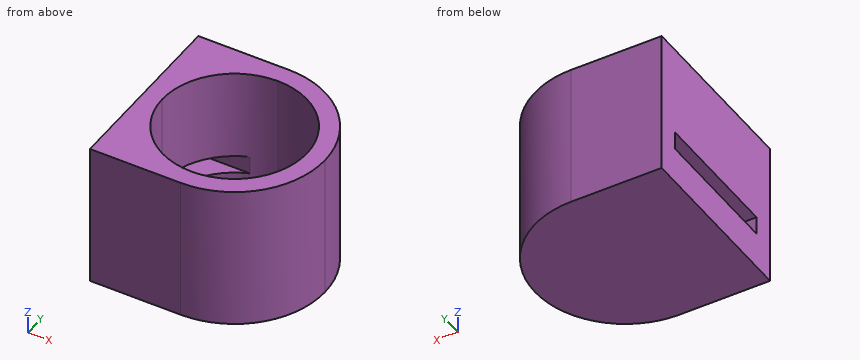
from build123d import *

# Parameters (mm, degrees)
F1_DEPTH = 25.4
F2_R     = 12.7
F3_DEPTH = 3.175
F5_DEPTH = 12.7


with BuildPart() as f1:
    # F0 (on Top) → F1 (new body)
    with BuildSketch(Plane.XY):
        with BuildLine():
            ThreePointArc((-15.875, 0), (-11.2253201513, 11.2253201513), (0, 15.875))
            Line((0, 15.875), (-15.875, 15.875))
            Line((-15.875, 15.875), (-15.875, 0))
        make_face()
        with BuildLine():
            Line((-15.875, -15.875), (0, -15.875))
            ThreePointArc((0, -15.875), (-11.2253201513, -11.2253201513), (-15.875, 0))
            Line((-15.875, 0), (-15.875, -15.875))
        make_face()
        with BuildLine():
            Line((0, -15.875), (0, -12.7))
            ThreePointArc((0, -12.7), (-8.9802561211, -8.9802561211), (-12.7, 0))
            Line((-12.7, 0), (-15.875, 0))
            ThreePointArc((-15.875, 0), (-11.2253201513, -11.2253201513), (0, -15.875))
        make_face()
        with BuildLine():
            ThreePointArc((-12.7, 0), (-8.9802561211, 8.9802561211), (0, 12.7))
            Line((0, 12.7), (0, 15.875))
            ThreePointArc((0, 15.875), (-11.2253201513, 11.2253201513), (-15.875, 0))
            Line((-15.875, 0), (-12.7, 0))
        make_face()
        with BuildLine():
            ThreePointArc((0, 12.7), (8.9802561211, 8.9802561211), (12.7, 0))
            ThreePointArc((12.7, 0), (8.9802561211, -8.9802561211), (0, -12.7))
            Line((0, -12.7), (0, -15.875))
            ThreePointArc((0, -15.875), (11.2253201513, -11.2253201513), (15.875, 0))
            ThreePointArc((15.875, 0), (11.2253201513, 11.2253201513), (0, 15.875))
            Line((0, 15.875), (0, 12.7))
        make_face()
    extrude(amount=F1_DEPTH)

    # F2 (on face) → F3 (join)
    with BuildSketch(Plane(origin=(0, 0, 0), x_dir=(1, 0, 0), z_dir=(0, 0, -1))):
        with BuildLine():
            Line((-15.875, 15.875), (-15.875, -15.875))
            Line((-15.875, -15.875), (0, -15.875))
            ThreePointArc((0, -15.875), (15.875, 0), (0, 15.875))
            Line((0, 15.875), (-15.875, 15.875))
        make_face()
        Circle(F2_R, mode=Mode.SUBTRACT)
        Circle(F2_R)
    extrude(amount=-F3_DEPTH)

    # F4 (on face) → F5 (cut)
    with BuildSketch(Plane(origin=(-15.875, 0, 0), x_dir=(0, -1, 0), z_dir=(-1, 0, 0))):
        Polygon((0, 6.35), (0, 9.525), (-7.9375, 9.525), (-11.90625, 9.525), (-11.90625, 6.35), (-7.9375, 6.35), align=None)
        Polygon((7.9375, 9.525), (0, 9.525), (0, 6.35), (7.9375, 6.35), (11.90625, 6.35), (11.90625, 9.525), align=None)
    extrude(amount=-F5_DEPTH, mode=Mode.SUBTRACT)


solid = f1.part
For this review, take the finished solid that the model builds, in its own axes (mm). Round coordinates to 2 decimals unless told otherwise and drop trailing zeros. Write each loop counter-clockwise with the first axis right and the second up, starting at its lowest first coordinate (ties: lowest second). Pieces come first, ordered by that corner, then holes. Notation, with made-up numbers: M 57,7.5 L 85,7.5 A9 cw 85,16.5 Z; hole C -16,-4 d3. An arc over 180 degrees is marked long. Write item = value, one per line. Start each with the question number.
(1) Clearance check with a flat-ended pin moving along its axis: pin 1 Ø1 at (x, z) = (6.5, 13.5) entering from -Y. State where the tip first meets the part, or that it passes through.
(2) For line 1 along Z through (x, y) = (5.5, 4.5) (3 decimals); line 2 along X through (y, z) = (4, 24) (3 decimals); line 3 along Y through (x, z) = (-6, 24) (3 decimals), list the stretches that pass through material, from the lowest coordinate up.
(3) We need section D-D (x = 8). Give the boundary of the cut face in (y, z) (3 decimals).
(4) We need section C-C (z = 8.25). Give the boundary of the cut face in (x, y) (3 decimals).
(5) We need section A-A (z = 20). Give the boundary of the cut face in (x, y) (3 decimals), then the cut area to 3 significant figures.
(6) We need section B-B (y = -4.5). Give the boundary of the cut face in (x, z) (3 decimals), then the cut area to 3 significant figures.
Results found:
q1.pin_1 = -14.7
q2.line_1 = 0 to 3.175
q2.line_2 = -15.875 to -12.054, 12.054 to 15.363
q2.line_3 = -15.875 to -11.193, 11.193 to 15.875
q3.outline = M -13.712,0 L 13.712,0 L 13.712,25.4 L 9.864,25.4 L 9.864,3.175 L -9.864,3.175 L -9.864,25.4 L -13.712,25.4 Z
q4.outline = M -15.875,-15.875 L 0,-15.875 A15.875 ccw 0,15.875 L -15.875,15.875 L -15.875,11.906 L -4.419,11.906 A12.7 cw long -4.419,-11.906 L -15.875,-11.906 Z
q5.outline = M -15.875,-15.875 L 0,-15.875 A15.875 ccw 0,15.875 L -15.875,15.875 Z; hole C 0,0 d25.4
q5.area = 393 mm²
q6.outline = M -15.875,0 L 15.224,0 L 15.224,25.4 L 11.876,25.4 L 11.876,3.175 L -11.876,3.175 L -11.876,6.35 L -15.875,6.35 Z; M -15.875,9.525 L -11.876,9.525 L -11.876,25.4 L -15.875,25.4 Z
q6.area = 249 mm²
